from build123d import *

# Parameters (mm, degrees)
SKICA1_W                                          = 75
SKICA1_H                                          = 110
SKICA1_W_2                                        = 35
SKICA1_H_2                                        = 70
P_IDAT_VYSUNUT_M1_DEPTH                           = 2.5
SKICA2_W                                          = 75
SKICA2_H                                          = 110
SKICA2_W_2                                        = 70
SKICA2_H_2                                        = 105
P_IDAT_VYSUNUT_M2_DEPTH                           = 15
P_IDAT_VYSUNUT_M3_REACH                           = 94.669
SKICA4_W                                          = 35
SKICA4_H                                          = 49.5
P_IDAT_VYSUNUT_M4_DEPTH                           = 2.5
SKICA5_W                                          = 70
SKICA5_H                                          = 2
P_IDAT_VYSUNUT_M5_DEPTH                           = 2
P_IDAT_VYSUNUT_M7_REACH                           = 94.669
KU_ELOV_ZAHLOUBEN_PRO_M4_ROUBU_SE_Z_P_D           = 4.5
KU_ELOV_ZAHLOUBEN_PRO_M4_ROUBU_SE_Z_P_CSINK_D     = 9.4
KU_ELOV_ZAHLOUBEN_PRO_M4_ROUBU_SE_Z_P_CSINK_ANGLE = 90
KU_ELOV_ZAHLOUBEN_PRO_M4_ROUBU_SE_2_A_COUNT       = 2
KU_ELOV_ZAHLOUBEN_PRO_M4_ROUBU_SE_2_A_PITCH       = 50
D_RY_PRO_KOL_K_VELIKOST_MM1_D                     = 3.9
D_RY_PRO_KOL_K_VELIKOST_MM1_DEPTH                 = 4
SKICA19_W                                         = 30
SKICA19_H                                         = 25
ODEBRAT_VYSUNUT_M1_DEPTH                          = 69.239931365
ODEBRAT_VYSUNUT_M4_DEPTH                          = 10
SKICA21_W                                         = 15
SKICA21_H                                         = 10
P_IDAT_VYSUNUT_M8_DEPTH                           = 2.5
V_LCOV_ZAHLOUBEN_PRO_M3_ROUBY_S_VNIT_D            = 3.4
V_LCOV_ZAHLOUBEN_PRO_M3_ROUBY_S_VNIT_DEPTH        = 5
V_LCOV_ZAHLOUBEN_PRO_M3_ROUBY_S_VNIT_CBORE_D      = 3.9
V_LCOV_ZAHLOUBEN_PRO_M3_ROUBY_S_VNIT_CBORE_DEPTH  = 4


with BuildPart() as part:
    # Skica1 → Přidat vysunutím1 (new body)
    with BuildSketch(Plane.XY):
        Rectangle(SKICA1_W, SKICA1_H)
        Rectangle(SKICA1_W_2, SKICA1_H_2, mode=Mode.SUBTRACT)
    extrude(amount=P_IDAT_VYSUNUT_M1_DEPTH)

    # Skica2 → Přidat vysunutím2 (add)
    with BuildSketch(Plane.XY.offset(2.5)):
        Rectangle(SKICA2_W, SKICA2_H)
        Rectangle(SKICA2_W_2, SKICA2_H_2, mode=Mode.SUBTRACT)
    extrude(amount=P_IDAT_VYSUNUT_M2_DEPTH)

    # Skica3 → Přidat vysunutím3 (add, up to next)
    with BuildSketch(Plane.ZY.offset(-35), mode=Mode.PRIVATE) as p_idat_vysunut_m3_sk1:
        Polygon((2.5, -52.5), (2.5, 14.5), (8.361740456, -52.5), align=None)
    p_idat_vysunut_m3_tool1 = extrude(p_idat_vysunut_m3_sk1.sketch, amount=P_IDAT_VYSUNUT_M3_REACH, mode=Mode.PRIVATE) - part.part
    add(p_idat_vysunut_m3_tool1.solids().sort_by_distance((35, -30.166667, 4.453913))[0])

    # Skica4 → Přidat vysunutím4 (add)
    with BuildSketch(Plane(origin=(0, 0, 2.5), x_dir=(-1, 0, 0), z_dir=(0, 0, -1))):
        with Locations((0, -10.25)):
            Rectangle(SKICA4_W, SKICA4_H)
    extrude(amount=P_IDAT_VYSUNUT_M4_DEPTH)

    # Skica5 → Přidat vysunutím5 (add)
    with BuildSketch(Plane(origin=(0, 0.327204013, 3.739958979), x_dir=(1, 0, 0), z_dir=(0, 0.08715574274765159, 0.9961946980917462))):
        with Locations((0, -40.02899535)):
            Rectangle(SKICA5_W, SKICA5_H)
    extrude(amount=P_IDAT_VYSUNUT_M5_DEPTH)

    # Skica9 → Přidat vysunutím7 (add, up to next)
    with BuildSketch(Plane.ZY.offset(-35), mode=Mode.PRIVATE) as p_idat_vysunut_m7_sk1:
        Polygon((9.308260939, -52.5), (9.308260939, -40.371352137), (7.315871543, -40.545663623), (8.361740456, -52.5), align=None)
    p_idat_vysunut_m7_tool1 = extrude(p_idat_vysunut_m7_sk1.sketch, amount=P_IDAT_VYSUNUT_M7_REACH, mode=Mode.PRIVATE) - part.part
    add(p_idat_vysunut_m7_tool1.solids().sort_by_distance((35, -45.761665, 8.543512))[0])

    # Ku_elov_ zahlouben_ pro M4 _roubu se z_p (through all)
    with Locations(Plane.XY.offset(9.308260939)):
        with Locations((25, -46.435676069), (-25, -46.435676069)):
            CounterSinkHole(KU_ELOV_ZAHLOUBEN_PRO_M4_ROUBU_SE_Z_P_D / 2, KU_ELOV_ZAHLOUBEN_PRO_M4_ROUBU_SE_Z_P_CSINK_D / 2, counter_sink_angle=KU_ELOV_ZAHLOUBEN_PRO_M4_ROUBU_SE_Z_P_CSINK_ANGLE)

    # Skica15 → Ku_elov_ zahlouben_ pro M4 _roubu se 2 (revolve, cut)
    with BuildSketch(Plane(origin=(25, 42.5, 2.5), x_dir=(0, -1, 0), z_dir=(1, 0, 0))):
        Polygon((0, 0), (0, 2.5), (2.25, 2.5), (2.25, 2.45), (4.7, 0), align=None)
    ku_elov_zahlouben_pro_m4_roubu_se_2 = revolve(axis=Axis((25, 42.5, 8.85), (0, 0, -1)), mode=Mode.SUBTRACT)

    # Ku_elov_ zahlouben_ pro M4 _roubu se 2 a: Ku_elov_ zahlouben_ pro M4 _roubu se 2 ×2
    with Locations(*[(-i * KU_ELOV_ZAHLOUBEN_PRO_M4_ROUBU_SE_2_A_PITCH, 0, 0) for i in range(1, KU_ELOV_ZAHLOUBEN_PRO_M4_ROUBU_SE_2_A_COUNT)]):
        add(ku_elov_zahlouben_pro_m4_roubu_se_2, mode=Mode.SUBTRACT)

    # Díry pro kolík, velikost mm1
    with Locations(Plane(origin=(0, 0.327204013, 3.739958979), x_dir=(1, 0, 0), z_dir=(0, 0.08715574274765159, 0.9961946980917462))):
        with Locations((32, -14.02899535), (-32, -14.02899535)):
            Hole(D_RY_PRO_KOL_K_VELIKOST_MM1_D / 2, depth=D_RY_PRO_KOL_K_VELIKOST_MM1_DEPTH)

    # Skica19 → Odebrat vysunutím1 (cut, through all)
    with BuildSketch(Plane(origin=(0, 0.327204013, 3.739958979), x_dir=(1, 0, 0), z_dir=(0, 0.08715574274765159, 0.9961946980917462))):
        with Locations((0, -12.401030792)):
            Rectangle(SKICA19_W, SKICA19_H)
    extrude(amount=-ODEBRAT_VYSUNUT_M1_DEPTH, mode=Mode.SUBTRACT)

    # Skica20 → Odebrat vysunutím4 (cut)
    with BuildSketch(Plane.XZ.offset(55)):
        Polygon((0, 9.5), (-20, 9.5), (-20, 17.5), (20, 17.5), (20, 9.5), align=None)
    extrude(amount=-ODEBRAT_VYSUNUT_M4_DEPTH, mode=Mode.SUBTRACT)

    # Skica21 → Přidat vysunutím8 (add)
    with BuildSketch(Plane(origin=(-35, 0, 0), x_dir=(0, 0, -1), z_dir=(1, 0, 0))):
        Polygon((-7.141560058, -38.553274227), (-6.273319169, -28.629235462), (-17.5, -27.64702816), (-17.5, -37.64702816), align=None)
        with Locations((-10, 42.5)):
            Rectangle(SKICA21_W, SKICA21_H)
    p_idat_vysunut_m8 = extrude(amount=P_IDAT_VYSUNUT_M8_DEPTH)

    # Zrcadlit1: Přidat vysunutím8 across plane
    add(p_idat_vysunut_m8.mirror(Plane(origin=(0, 0, 0), x_dir=(0, 0, 1), z_dir=(1, 0, 0))))

    # Válcové zahloubení pro M3 šrouby s vnitřním šestihranem1
    with Locations(Plane(origin=(-32.5, 0, 0), x_dir=(0, 0, -1), z_dir=(1, 0, 0))):
        with Locations((-13.5, 42.5), (-13.515221208, -32.995651131)):
            v_lcov_zahlouben_pro_m3_rouby_s_vnit = CounterBoreHole(V_LCOV_ZAHLOUBEN_PRO_M3_ROUBY_S_VNIT_D / 2, V_LCOV_ZAHLOUBEN_PRO_M3_ROUBY_S_VNIT_CBORE_D / 2, V_LCOV_ZAHLOUBEN_PRO_M3_ROUBY_S_VNIT_CBORE_DEPTH, depth=V_LCOV_ZAHLOUBEN_PRO_M3_ROUBY_S_VNIT_DEPTH)

    # Zrcadlit2: Válcové zahloubení pro M3 šrouby s vnitřním šestihranem1 across plane
    add(v_lcov_zahlouben_pro_m3_rouby_s_vnit.mirror(Plane(origin=(0, 0, 0), x_dir=(0, 0, 1), z_dir=(1, 0, 0))), mode=Mode.SUBTRACT)


solid = part.part
Can you work these out from the model? Positions are in its coordinate system, mm. A direction names the side the tool comes from. Coordinates: 2 decimals unless noted, no trailing zeros. Write each loop counter-clockwise with the first axis right and the second up, starting at its lowest first coordinate (ties: lowest second). Pieces come first, ordered by that corner, then holes. Notation, with made-up numbers: (51, 88) -> (98, 88) arc R8 ccw to (98, 95) -> close; hole circle Ø5 at (63, 63.25). An arc over 180 degrees is marked (long way). Answer as CSV lines item,"result".
1) If we section it at C-C on x = -13: Please give me the cut outline in (y, z), then the cut area to 3 significant figures.
Check result:
outline,"(-55, 0) -> (-25, 0) -> (-24.48, 5.91) -> (-38.55, 7.14) -> (-38.38, 9.13) -> (-40.37, 9.31) -> (-52.5, 9.31) -> (-52.5, 9.5) -> (-55, 9.5) -> close; (0.1, 0) -> (14.5, 0) -> (14.5, 2.5) -> (0.43, 3.73) -> close; (35, 0) -> (55, 0) -> (55, 17.5) -> (52.5, 17.5) -> (52.5, 2.5) -> (35, 2.5) -> close"
area,"376 mm²"
2) If I drill on line 1 (Y direction, x = -35.55, z = 13.5); line 2 (X direction, y = -14, z = 1.5); line 3 (X direction, y = -38, z = 11.5), over which ranges is the centre line in solid material (lowest first)? Write a range as from..to.
Check result:
line 1,"-55..-34.95, -31.05..40.55, 44.45..55"
line 2,"-37.5..-33.95, -30.05..-15, 15..30.05, 33.95..37.5"
line 3,"-37.5..-32.5, 32.5..37.5"
3) Will these pins go through, and if not, where does the flat tip stop? P1, Ø4, axis at x = -11, y = 37, coming from the +Z side; P2, Ø3, axis at x = 12.5, z = 15.5, coming from the -Y side.
Check result:
P1,"z = 2.5"
P2,"y = 52.5"
4) If we section it at D-D on y = 12: Please give me the cut outline in (x, z), then the cut area to 3 significant figures.
Check result:
outline,"(-37.5, 0) -> (37.5, 0) -> (37.5, 17.5) -> (35, 17.5) -> (35, 2.72) -> (-35, 2.72) -> (-35, 17.5) -> (-37.5, 17.5) -> close"
area,"278 mm²"
5) If we mould it in two halves opening along Y, with no side actions, what happens to faces 1 (the flat face through (32.5, 43, 10)), 2 (the flat face through (-1, 55, 9)), 3 (the flat face through (-36, 8, 17.5))? For each: +Y half, -Y half, draft (parallel to the pull), parting line (faces both ways), or undercut.
Check result:
face 1,"undercut"
face 2,"+Y half"
face 3,"draft"
6) If we section it at B-B on y = 33: Please give me the cut outline in (x, z), then the cut area to 3 significant figures.
Check result:
outline,"(-37.5, 0) -> (-17.5, 0) -> (-17.5, 2.5) -> (-35, 2.5) -> (-35, 17.5) -> (-37.5, 17.5) -> close; (17.5, 0) -> (37.5, 0) -> (37.5, 17.5) -> (35, 17.5) -> (35, 2.5) -> (17.5, 2.5) -> close"
area,"175 mm²"
7) On a 3-axis mill with a long thin cutter (end or side, diameter ignored), from which of +Z, -Z, +X, -X, +Y, -Y can I reach the whole of each face in a straight line? I mean faces 4 (the flat face through (-1, -55, 7)), 5 (the flat face through (34, 37.5, 10)), 6 (the cylindrical face through (-26.04, -48.43, 3.38)), 7 (the cylindrical face through (-34.472, 41.313, 15.047)), 8 (the flat face through (-0.21, -24.734, 2.996)). Say none if no direction works.
Check result:
face 4,"+Z, -Z, +X, -X, -Y"
face 5,"+Z"
face 6,"+Z, -Z"
face 7,"none"
face 8,"-Z"
8) If we section it at A-A on x = -25: Please give me the cut outline in (y, z).
Check result:
outline,"(-55, 0) -> (-48.69, 0) -> (-48.69, 6.86) -> (-51.14, 9.31) -> (-52.5, 9.31) -> (-52.5, 17.5) -> (-55, 17.5) -> close; (-44.19, 0) -> (40.25, 0) -> (40.25, 0.05) -> (37.8, 2.5) -> (14.5, 2.5) -> (-38.55, 7.14) -> (-38.38, 9.13) -> (-40.37, 9.31) -> (-41.74, 9.31) -> (-44.19, 6.86) -> close; (44.75, 0) -> (55, 0) -> (55, 17.5) -> (52.5, 17.5) -> (52.5, 2.5) -> (47.2, 2.5) -> (44.75, 0.05) -> close"
